Autodesk Inventor part; units mm, degrees
ref_plane "YZ Plane" through (0, 0, 0) normal (1, 0, 0) x (0, 1, 0)
ref_plane "XZ Plane" through (0, 0, 0) normal (0, 1, 0) x (-1, 0, 0)
ref_plane "XY Plane" through (0, 0, 0) normal (0, 0, 1) x (1, 0, 0)
sketch "Sketch1" plane through (0, 0, 0) normal (0, 0, 1) x (1, 0, 0)
  line L0 (177.8, 0) -> (177.8, 152.4)
  line L1 (0, 152.4) -> (0, 0)
  line L2 (152.4, 152.4) -> (152.4, 155.575)
  line L3 (152.4, 155.575) -> (25.4, 155.575)
  line L4 (25.4, 155.575) -> (25.4, 152.4)
  line L5 (0, 152.4) -> (25.4, 152.4)
  line L6 (152.4, 152.4) -> (177.8, 152.4)
  line L7 (152.4, 0) -> (152.4, -3.175)
  line L8 (152.4, -3.175) -> (25.4, -3.175)
  line L9 (25.4, -3.175) -> (25.4, 0)
  line L10 (0, 0) -> (25.4, 0)
  line L11 (152.4, 0) -> (177.8, 0)
  dimension "d0" = 152.4
  dimension "d1" = 177.8
  dimension "d18" = 25.4
  dimension "d19" = 25.4
  dimension "d20" = 3.175
extrude "Extrusion3" add sketch "Sketch1" along normal blind 3.175
sketch "Sketch2" plane through (0, 0, 3.175) normal (0, 0, 1) x (1, 0, 0)
  line L0 (0, 152.4) -> (25.4, 152.4)
  line L1 (0, 0) -> (0, 152.4)
  line L2 (25.4, 0) -> (0, 0)
  line L3 (177.8, 0) -> (152.4, 0)
  line L4 (152.4, 152.4) -> (177.8, 152.4)
  line L5 (25.4, 152.4) -> (25.4, 155.575)
  line L6 (12.7, 152.4) -> (12.7, 139.7) construction
  line L7 (12.7, 139.7) -> (12.7, 114.3) construction
  line L8 (12.7, 114.3) -> (12.7, 88.9) construction
  line L9 (12.7, 88.9) -> (12.7, 63.5) construction
  line L10 (12.7, 63.5) -> (12.7, 38.1) construction
  line L11 (12.7, 38.1) -> (12.7, 12.7) construction
  line L12 (12.7, 12.7) -> (12.7, 0) construction
  circle A0 centre (12.7, 139.7) radius 2.3813
  circle A1 centre (12.7, 114.3) radius 2.3813
  circle A2 centre (12.7, 88.9) radius 2.3813
  circle A3 centre (12.7, 63.5) radius 2.3813
  circle A4 centre (12.7, 38.1) radius 2.3813
  circle A5 centre (12.7, 12.7) radius 2.3813
  line L13 (165.1, 152.4) -> (165.1, 139.7) construction
  line L14 (165.1, 139.7) -> (165.1, 114.3) construction
  line L15 (165.1, 114.3) -> (165.1, 88.9) construction
  line L16 (165.1, 88.9) -> (165.1, 63.5) construction
  line L17 (165.1, 63.5) -> (165.1, 38.1) construction
  line L18 (165.1, 38.1) -> (165.1, 12.7) construction
  line L19 (165.1, 12.7) -> (165.1, 0) construction
  circle A6 centre (165.1, 139.7) radius 2.3813
  circle A7 centre (165.1, 114.3) radius 2.3813
  circle A8 centre (165.1, 88.9) radius 2.3813
  circle A9 centre (165.1, 63.5) radius 2.3813
  circle A10 centre (165.1, 38.1) radius 2.3813
  circle A11 centre (165.1, 12.7) radius 2.3813
  dimension "d26" = 12.7
  dimension "d27" = 25.4
  dimension "d28" = 4.7625
  dimension "d29" = 12.7
  dimension "d30" = 25.4
  dimension "d31" = 4.7625
extrude "Extrusion4" cut sketch "Sketch2" against normal up to next
sketch "Sketch3" plane through (0, 0, 3.175) normal (0, 0, 1) x (1, 0, 0)
  line L0 (0, 0) -> (0, 152.4)
  line L1 (25.4, 0) -> (0, 0)
  circle A0 centre (76.2, 127) radius 3.175
  circle A1 centre (76.2, 12.7) radius 3.175
  dimension "d34" = 76.2
  dimension "d35" = 76.2
  dimension "d36" = 114.3
  dimension "d37" = 12.7
  dimension "d38" = 6.35
  dimension "d39" = 6.35
extrude "Extrusion5" cut sketch "Sketch3" against normal up to next
sketch "Sketch4" plane through (0, 0, 3.175) normal (0, 0, 1) x (1, 0, 0)
  circle A0 centre (76.2, 127) radius 3.175
  line L0 (177.8, 0) -> (152.4, 0)
  line L1 (177.8, 152.4) -> (177.8, 0)
  line L2 (152.4, 152.4) -> (177.8, 152.4)
  line L3 (92.075, 139.7) -> (142.875, 139.7)
  line L4 (146.05, 136.525) -> (146.05, 15.875)
  line L5 (142.875, 12.7) -> (92.075, 12.7)
  line L6 (88.9, 15.875) -> (88.9, 136.525)
  arc A1 (92.075, 139.7) -> (88.9, 136.525) centre (92.075, 136.525) ccw
  arc A2 (146.05, 136.525) -> (142.875, 139.7) centre (142.875, 136.525) ccw
  arc A3 (142.875, 12.7) -> (146.05, 15.875) centre (142.875, 15.875) ccw
  arc A4 (88.9, 15.875) -> (92.075, 12.7) centre (92.075, 15.875) ccw
  dimension "d42" = 12.7
  dimension "d43" = 31.75
  dimension "d44" = 12.7
  dimension "d45" = 12.7
  dimension "d46" = 3.175
extrude "Extrusion6" cut sketch "Sketch4" against normal up to next contours L3 A2 L4 A3 L5 A4 L6 A1
sketch "Sketch5" plane through (0, 0, 3.175) normal (0, 0, 1) x (1, 0, 0)
  line L0 (25.4, 155.575) -> (152.4, 155.575)
  line L1 (152.4, 155.575) -> (152.4, 152.4)
  line L2 (152.4, 152.4) -> (25.4, 152.4)
  line L3 (25.4, 152.4) -> (25.4, 155.575)
  line L4 (25.4, -3.175) -> (152.4, -3.175)
  line L5 (152.4, -3.175) -> (152.4, 0)
  line L6 (152.4, 0) -> (25.4, 0)
  line L7 (25.4, 0) -> (25.4, -3.175)
extrude "Extrusion7" add sketch "Sketch5" along normal blind 6.35
properties part number "DriveTrain_MotorMount" material "Aluminum-6061"
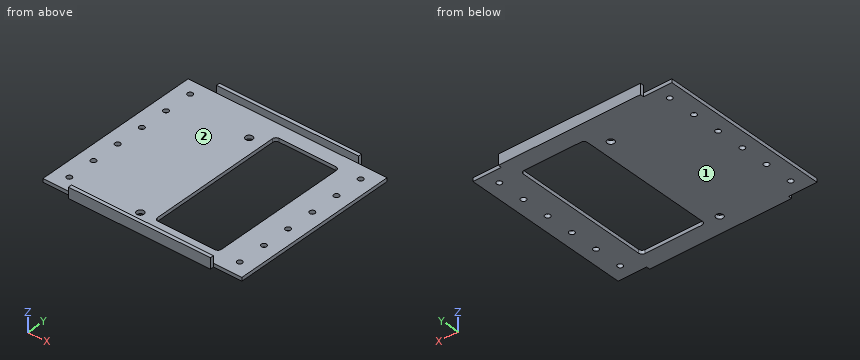
Build history of the part. All positions in model axes, mm. Face numbers are marked on the shaded views. Round coordinates to 2 decimals unless told otherwise and drop trailing zeros. Loops run counter-clockwise (first coordinate to the right, second up) from the corner with the lowest first, then second, coordinate; pieces in that order, holes last.
Item 1: Saw through at A-A (y = 38.1). List the corners of the cut face in (x, z) (3 decimals).
Item 2: Saw through at D-D (z = 8). List the corners of the cut face in (x, y) (3 decimals).
Item 3: Saw through at C-C (y = 127). List the corners of the cut face in (x, z) (3 decimals).
Item 4: Saw through at B-B (x = 12.7). List the corners of the cut face in (y, z) (3 decimals), then the cut area to 3 significant figures.
Item 5: Pin check, flat tips, straight feed: P1, Ø2.5, axis at y = 154.5, z = 7, coming from the -X side; P2, Ø4.5, axis at x = 12.7, y = 38.1, coming from the +Z side; P3, Ø3.5, axis at y = 154, z = 5.5, coming from the +X side; P4, Ø2, axis at x = 25, y = 128.5, coming from the +Z side (3 decimals). Stop position of each tip, or through.
Item 6: Drill centre lines: line 1 along X through (y, z) = (140, 2.5); line 2 along Y through (x, z) = (116, 5.75) (3 decimals); line 3 along Z through (x, y) = (79.5, 136.5) (3 decimals). Where is each one in solid material? Low to high.
Item 7: Two-plate mould, pull along Y, no slides. Class the marked faces 1 and 2: released by +Y, released by -Y, zero draft, split by the parting line, or undercut.
Worked answers:
1. outline: (0, 0) - (10.319, 0) - (10.319, 3.175) - (0, 3.175) - close; (15.081, 0) - (88.9, 0) - (88.9, 3.175) - (15.081, 3.175) - close; (146.05, 0) - (162.719, 0) - (162.719, 3.175) - (146.05, 3.175) - close; (167.481, 0) - (177.8, 0) - (177.8, 3.175) - (167.481, 3.175) - close
2. outline: (25.4, -3.175) - (152.4, -3.175) - (152.4, 0) - (25.4, 0) - close; (25.4, 152.4) - (152.4, 152.4) - (152.4, 155.575) - (25.4, 155.575) - close
3. outline: (0, 0) - (73.025, 0) - (73.025, 3.175) - (0, 3.175) - close; (79.375, 0) - (88.9, 0) - (88.9, 3.175) - (79.375, 3.175) - close; (146.05, 0) - (177.8, 0) - (177.8, 3.175) - (146.05, 3.175) - close
4. outline: (0, 0) - (10.319, 0) - (10.319, 3.175) - (0, 3.175) - close; (15.081, 0) - (35.719, 0) - (35.719, 3.175) - (15.081, 3.175) - close; (40.481, 0) - (61.119, 0) - (61.119, 3.175) - (40.481, 3.175) - close; (65.881, 0) - (86.519, 0) - (86.519, 3.175) - (65.881, 3.175) - close; (91.281, 0) - (111.919, 0) - (111.919, 3.175) - (91.281, 3.175) - close; (116.681, 0) - (137.319, 0) - (137.319, 3.175) - (116.681, 3.175) - close; (142.081, 0) - (152.4, 0) - (152.4, 3.175) - (142.081, 3.175) - close
4. area: 393 mm2
5. P1: stops at x = 25.4
5. P2: passes through
5. P3: stops at x = 152.4
5. P4: stops at z = 3.175
6. line 1: x = 0 to 10.34, 15.06 to 162.74, 167.46 to 177.8
6. line 2: y = -3.175 to 0, 152.4 to 155.575
6. line 3: z = 0 to 3.175
7. face 1: zero draft
7. face 2: undercut
